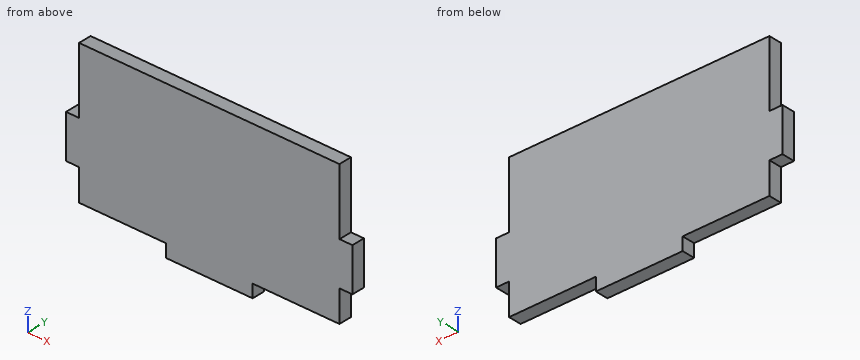
```python
from build123d import *

# Parameters (mm, degrees)
SKETCH2_W           = 60
SKETCH2_H           = 35.5
BOSS_EXTRUDE1_DEPTH = 3
SKETCH3_W           = 3
SKETCH3_H           = 10
BOSS_EXTRUDE2_DEPTH = 3
SKETCH4_W           = 20
SKETCH4_H           = 3
CUT_EXTRUDE2_DEPTH  = 3


with BuildPart() as part:
    # Sketch2 → Boss-Extrude1 (new body)
    with BuildSketch(Plane(origin=(0, 0, 0), x_dir=(1, 0, 0), z_dir=(0, 1, 0))):
        Rectangle(SKETCH2_W, SKETCH2_H)
    extrude(amount=BOSS_EXTRUDE1_DEPTH)

    # Sketch3 → Boss-Extrude2 (add)
    with BuildSketch(Plane(origin=(0, 0, 0), x_dir=(1, 0, 0), z_dir=(0, 1, 0))):
        with Locations((-31.5, 2.5)):
            Rectangle(SKETCH3_W, SKETCH3_H)
        with Locations((31.5, 2.5)):
            Rectangle(SKETCH3_W, SKETCH3_H)
    extrude(amount=BOSS_EXTRUDE2_DEPTH)

    # Sketch4 → Cut-Extrude2 (cut)
    with BuildSketch(Plane(origin=(0, 3, 0), x_dir=(1, 0, 0), z_dir=(0, 1, 0))):
        with Locations((-20, 16.25)):
            Rectangle(SKETCH4_W, SKETCH4_H)
        with Locations((20, 16.25)):
            Rectangle(SKETCH4_W, SKETCH4_H)
    extrude(amount=-CUT_EXTRUDE2_DEPTH, mode=Mode.SUBTRACT)


solid = part.part
```
CAD build for the part. Positions are in the model's coordinates, mm. Give positions to 0.01 mm unless a question says otherwise; leave off trailing zeros. Write each loop counter-clockwise with the first axis right and the second up, starting at its lowest first coordinate (ties: lowest second). Pieces come first, ordered by that corner, then holes. Notation, with made-up numbers: M 82,-25.5 L 128,-25.5 A22 ccw 128,9.5 Z; hole C -27.5,32.5 d2. An arc over 180 degrees is marked long. Return JSON: item names as keys, results as strings. Group by question number.
(1) Band-saw the part on C-C (x = 22). Give the cut face in (y, z).
(2) Flat gauge pins, fed straight in: pin 1 Ø1.5 at (x, y) = (-31, 1) entering from -Z; pin 2 Ø1.5 at (y, z) = (1, -16) entering from -X; pin 3 Ø1.5 at (x, y) = (-23.5, 2) entering from -Z. Where does each tip first touch, or does it go through?
(3) Drill centre lines: L1, parallel to X at y = 1.6, z = -8; L2, parallel to Z at x = 15, y = 2.5; L3, parallel to Z at x = 30.5, y = 2.05. Where is each one in solid material? Low to high. Write a range as [from, to].
(4) Band-saw the part on A-A (y = 1.55). Give the cut face in (x, z).
(5) Band-saw the part on B-B (z = -13). Give the cut face in (x, y).
Entries:
{
 "1": {"outline": "M 0,-14.75 L 3,-14.75 L 3,17.75 L 0,17.75 Z"},
 "2": {"pin 1": "stops at z = -7.5", "pin 2": "stops at x = -10", "pin 3": "stops at z = -14.75"},
 "3": {"L1": "x = [-30, 30]", "L2": "z = [-14.75, 17.75]", "L3": "z = [-7.5, 2.5]"},
 "4": {"outline": "M -33,-7.5 L -30,-7.5 L -30,-14.75 L -10,-14.75 L -10,-17.75 L 10,-17.75 L 10,-14.75 L 30,-14.75 L 30,-7.5 L 33,-7.5 L 33,2.5 L 30,2.5 L 30,17.75 L -30,17.75 L -30,2.5 L -33,2.5 Z"},
 "5": {"outline": "M -30,0 L 30,0 L 30,3 L -30,3 Z"}
}
